Geometry: final body of the model. Coordinates: model frame, mm. A direction names the side the tool comes from. Round coordinates to 2 decimals unless told otherwise and drop trailing zeros. Loops run counter-clockwise (first coordinate to the right, second up) from the corner with the lowest first, then second, coordinate; pieces in that order, holes last. Notation, with made-up numbers: (69.5, -25) - (110.5, -25) arc R20 ccw to (110.5, 13) - close; hole circle Ø4 at (-1, 83). An arc over 180 degrees is marked (long way). Answer as a JSON object with one key per item and string values. Group by question number.
Item 1: Section B-B (z = -12.5). Return the cut outline in (x, y), plus the area to 3 significant figures.
Item 2: Draft query along X for faces 1 (the face through (11.49, -12.32, -41.53)), 2 (the face through (-5, -12, -37)), 3 (the face through (34.14, -12.32, 4.1)). Return one class per face: released by +X, released by -X, zero draft, split by the parting line, or undercut.
Item 3: First-contact query: pin 1 (12 mm diameter, centred on x = 31, y = -15.5, fed in from -Z); pin 2 (1 mm diameter, centred on y = -12.5, z = -19, fed in from +X); pin 3 (7.5 mm diameter, centred on y = -15, z = -56.5, fed in from +X). Flat tips, straight axial feed; report the tip coordinate or a pass-through.
Item 4: Section C-C (x = 20.5). Return the cut outline in (y, z).
Item 5: Section D-D (x = 9). Return the cut outline in (y, z), plus the area to 3 significant figures.
Item 6: Reachability of faces 4 (the face through (0, -12, -39)), 5 (the face through (15, -12, 0)), 6 (the face through (-4.1, -12.32, 4.14)) from +Z, -Z, +X, -X, +Y, -Y: full face, straight path, thin tool, end or side. Return the list, or none.
Item 7: Line query: line 1 (X direction, y = -6.75, z = -11); line 2 (Z direction, x = 28, y = -15.25); line 3 (Z direction, x = 22.5, y = -18.5). Output: solid intervals per line, ascending.
Item 8: Section A-A (y = -18.75). Return the cut outline in (x, z), plus the area to 3 significant figures.
```python
from build123d import *

# Parameters (mm, degrees)
F1_DEPTH    = 25
F2_T1_DEPTH = 40
F2_T3_DEPTH = 36.0263819839
F2_T5_DEPTH = 41.8333819759
F2_T7_DEPTH = 39.2479422715


# Not quite as in the source:
# - a fillet or chamfer that OpenCascade refuses, or shapes differently, is made with other operations: its cross-section is extruded or revolved along the edge and cut away or added


with BuildPart() as f1:
    # F0 (on Front) → F1 (new body)
    with BuildSketch(Plane.XZ):
        with BuildLine():
            Line((-5, -80), (0, -80))
            Line((0, -80), (0, 0))
            Line((0, 0), (30, 0))
            Line((30, 0), (30, -15.6914651025))
            ThreePointArc((30, -15.6914651025), (11.4304994047, -43.4285104275), (30, -71.1655557525))
            Line((30, -71.1655557525), (32.6106493124, -66.8210358224))
            ThreePointArc((32.6106493124, -66.8210358224), (16.4620002863, -42.1738982265), (35, -19.26968849))
            Line((35, -19.26968849), (35, 5))
            Line((35, 5), (-5, 5))
            Line((-5, 5), (-5, -80))
        make_face()
    extrude(amount=F1_DEPTH)

    # F2: fillet of radius 3 on 7 edges, made by hand

    # F2_s2 → F2_t1 (cut)
    with BuildSketch(Plane.XZ.offset(-7.5)):
        with BuildLine():
            ThreePointArc((35, 2), (34.1213203436, 4.1213203436), (32, 5))
            Line((32, 5), (35, 5))
            Line((35, 5), (35, 2))
        make_face()
        with BuildLine():
            ThreePointArc((-3, -80), (-0.8786796564, -79.1213203436), (0, -77))
            Line((0, -77), (0, -80))
            Line((0, -80), (-3, -80))
        make_face()
        with BuildLine():
            ThreePointArc((-2, -80), (-4.1213203436, -79.1213203436), (-5, -77))
            Line((-5, -77), (-5, -80))
            Line((-5, -80), (-2, -80))
        make_face()
        with BuildLine():
            ThreePointArc((-2, 5), (-4.1213203436, 4.1213203436), (-5, 2))
            Line((-5, 2), (-5, 5))
            Line((-5, 5), (-2, 5))
        make_face()
    extrude(amount=F2_T1_DEPTH, mode=Mode.SUBTRACT)

    # F2_s4 → F2_t3 (cut)
    with BuildSketch(Plane.XZ.offset(-5.513190992)):
        with BuildLine():
            ThreePointArc((33.0104106505, -19.8891369147), (34.4526752691, -18.7919490752), (35, -17.0644120932))
            Line((35, -17.0644120932), (35, -19.26968849))
            ThreePointArc((35, -19.26968849), (33.9987485172, -19.5586742582), (33.0104106505, -19.8891369147))
        make_face()
    extrude(amount=F2_T3_DEPTH, mode=Mode.SUBTRACT)

    # F2_s6 → F2_t5 (cut)
    with BuildSketch(Plane.XZ.offset(-8.416690988)):
        with BuildLine():
            ThreePointArc((30.8765859694, -69.7067825667), (31.1957188728, -67.3587557485), (29.7114248515, -65.5116101106))
            ThreePointArc((29.7114248515, -65.5116101106), (31.1401881693, -66.212484942), (32.6106493124, -66.8210358224))
            Line((32.6106493124, -66.8210358224), (30.8765859694, -69.7067825667))
        make_face()
    extrude(amount=F2_T5_DEPTH, mode=Mode.SUBTRACT)

    # F2_s8 → F2_t7 (cut)
    with BuildSketch(Plane.XZ.offset(-7.1239711357)):
        with BuildLine():
            ThreePointArc((27.4198994503, -69.9559130315), (29.6266357528, -70.1929626749), (31.39240951, -68.8483732652))
            Line((31.39240951, -68.8483732652), (30, -71.1655557525))
            ThreePointArc((30, -71.1655557525), (28.695579184, -70.5913859559), (27.4198994503, -69.9559130315))
        make_face()
    extrude(amount=F2_T7_DEPTH, mode=Mode.SUBTRACT)


solid = f1.part
```
Values:
{
 "1": {"outline": "(-5, -25) - (0, -25) - (0, 0) - (-5, 0) - close; (30, -25) - (35, -25) - (35, 0) - (30, 0) - close", "area": "250 mm^2"},
 "2": {"face 1": "undercut", "face 2": "released by -X", "face 3": "released by +X"},
 "3": {"pin 1": "stops at z = -70.3", "pin 2": "stops at x = 34.63", "pin 3": "stops at x = 22.94"},
 "4": {"outline": "(-25, -64.92) - (0, -64.92) - (0, -57.1) - (-25, -57.1) - close; (-25, -29.76) - (0, -29.76) - (0, -21.94) - (-25, -21.94) - close; (-25, 0) - (0, 0) - (0, 5) - (-25, 5) - close"},
 "5": {"outline": "(-25, 0) - (0, 0) - (0, 5) - (-25, 5) - close", "area": "125 mm^2"},
 "6": {"face 4": "-Z, +Y, -Y", "face 5": "+Y, -Y", "face 6": "+Z, -X, +Y, -Y"},
 "7": {"line 1": "x = -5 to 0, 30 to 35", "line 2": "z = -70.19 to -64.51, -22.34 to -16.6, 0 to 5", "line 3": "z = -66.7 to -59.76, -27.1 to -20.16, 0 to 5"},
 "8": {"outline": "(-5, -77) arc R3 ccw to (-2.5, -79.96) arc R3 ccw to (0, -77) - (0, 0) - (30, 0) - (30, -15.69) arc R30 ccw to (27.42, -69.96) arc R3 ccw to (31.1, -69.26) arc R3 ccw to (29.71, -65.51) arc R25 cw to (33.01, -19.89) arc R3 ccw to (35, -17.06) - (35, 2) arc R3 ccw to (32, 5) - (-2, 5) arc R3 ccw to (-5, 2) - close", "area": "1,010 mm^2"}
}
